from build123d import *

# Parameters (mm, degrees)
SKETCH1_W                      = 50
SKETCH1_H                      = 200
BOSS_EXTRUDE1_DEPTH            = 70
M6_CLEARANCE_HOLE1_D           = 6.6
M6_CLEARANCE_HOLE1_DEPTH       = 3.017159957
M6_CLEARANCE_HOLE1_CSINK_D     = 6.65
M6_CLEARANCE_HOLE1_CSINK_ANGLE = 100
M6_CLEARANCE_HOLE1_TIP         = 1.982840043
SKETCH5_R                      = 10
SKETCH5_R_2                    = 18.5
CUT_EXTRUDE1_DEPTH             = 40
M6_CLEARANCE_HOLE2_D           = 6.6
M6_CLEARANCE_HOLE2_CSINK_D     = 6.65
M6_CLEARANCE_HOLE2_CSINK_ANGLE = 100


with BuildPart() as part:
    # Sketch1 → Boss-Extrude1 (new body)
    with BuildSketch(Plane(origin=(0, 0, 0), x_dir=(1, 0, 0), z_dir=(0, 1, 0))):
        Rectangle(SKETCH1_W, SKETCH1_H)
    extrude(amount=BOSS_EXTRUDE1_DEPTH)

    # M6 Clearance Hole1
    with Locations(Plane(origin=(0, 0, 0), x_dir=(-1, 0, 0), z_dir=(0, -1, 0))):
        with Locations((0, 75), (0, 0), (0, -75)):
            CounterSinkHole(M6_CLEARANCE_HOLE1_D / 2, M6_CLEARANCE_HOLE1_CSINK_D / 2, depth=M6_CLEARANCE_HOLE1_DEPTH, counter_sink_angle=M6_CLEARANCE_HOLE1_CSINK_ANGLE)
            with Locations((0, 0, -(M6_CLEARANCE_HOLE1_DEPTH + M6_CLEARANCE_HOLE1_TIP / 2))):  # 118° drill point
                Cone(0, M6_CLEARANCE_HOLE1_D / 2, M6_CLEARANCE_HOLE1_TIP, mode=Mode.SUBTRACT)

    # Sketch5 → Cut-Extrude1 (cut)
    with BuildSketch(Plane.ZY.offset(25)):
        with Locations((-60, 40)):
            Circle(SKETCH5_R)
        with Locations((60, 40)):
            Circle(SKETCH5_R)
        with Locations((0, 40)):
            Circle(SKETCH5_R_2)
    extrude(amount=-CUT_EXTRUDE1_DEPTH, mode=Mode.SUBTRACT)

    # M6 Clearance Hole2 (through all)
    with Locations(Plane(origin=(0, 70, 0), x_dir=(1, 0, 0), z_dir=(0, 1, 0))):
        with Locations((-15, 40), (15, 40), (-15, -40), (15, -40)):
            CounterSinkHole(M6_CLEARANCE_HOLE2_D / 2, M6_CLEARANCE_HOLE2_CSINK_D / 2, counter_sink_angle=M6_CLEARANCE_HOLE2_CSINK_ANGLE)


solid = part.part
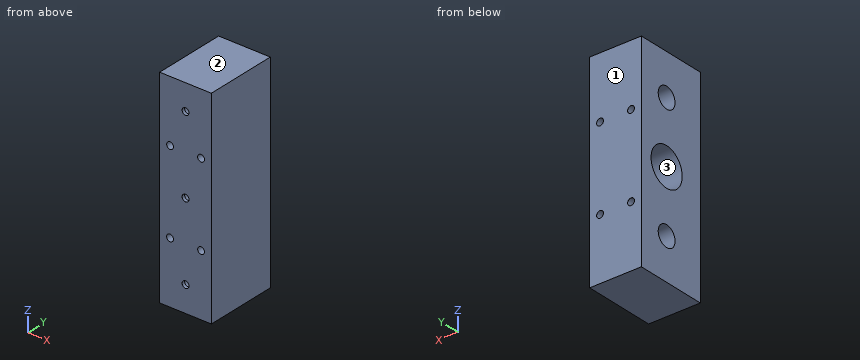
Work out the finished part from the listing and answer in its coordinate system (mm). Face numbers are marked on the shaded views. Give positions to 0.01 mm unless a question says otherwise; leave off trailing zeros. Write each loop counter-clockwise with the first axis right and the second up, starting at its lowest first coordinate (ties: lowest second). Pieces come first, ordered by that corner, then holes. Notation, with made-up numbers: M -4.75,80 L 46.25,80 A36 cw 46.25,119 Z; hole C 61.25,77.25 d4. An arc over 180 degrees is marked long. Answer as CSV lines item,"result".
Q1. Find the intervals of material crossed by probe 1 along X at (y, z) = (46, -40); probe 2 along Z at (x, y) = (0, 2); probe 3 along X at (y, z) = (63.5, -42), in increasing order. Write a range as [from, to].
A:
probe 1,"x = [-25, -18.3], [-11.7, 11.7], [18.3, 25]"
probe 2,"z = [-100, -78.3], [-71.7, -3.3], [3.3, 71.7], [78.3, 100]"
probe 3,"x = [-25, -17.62], [-12.38, 12.38], [17.62, 25]"
Q2. The mould has two halves that part along Z. Classify the marked faces 1, 2 and 3: +Z half, -Z half, draft (parallel to the pull), parting line (faces both ways), or undercut.
A:
face 1,"draft"
face 2,"+Z half"
face 3,"undercut"
Q3. A cutting plane is placed at A-A on z = -40. Write down the section's boundary in (x, y) (3 decimals).
A:
outline,"M -25,0 L -18.3,0 L -18.3,69.979 L -18.325,70 L -25,70 Z; M -11.7,0 L 11.7,0 L 11.7,69.979 L 11.675,70 L -11.675,70 L -11.7,69.979 Z; M 18.3,0 L 25,0 L 25,70 L 18.325,70 L 18.3,69.979 Z"
Q4. Given P1, Ø18, axis at y = 40, z = 60, coming from the -X side, flat-ended and moving along its own axis, determine where the tip first touches the part or whether it passes through.
A:
P1,"stops at x = 15"
Q5. A cutting plane is placed at D-D on x = -16. Count the separate pieces of the cut face and the enclosed holes in it, plus the area to 3 significant figures.
A:
separate pieces,"3"
enclosed holes,"3"
area,"11,400 mm²"
Q6. A cutting plane is placed at B-B on y = 40. Write down the section's boundary in (x, z), plus the area to 3 significant figures.
A:
outline,"M -25,-100 L 25,-100 L 25,100 L -25,100 L -25,70 L 15,70 L 15,50 L -25,50 L -25,18.5 L 15,18.5 L 15,-18.5 L -25,-18.5 L -25,-50 L 15,-50 L 15,-70 L -25,-70 Z; hole C -15,-40 d6.6; hole C -15,40 d6.6; hole C 15,-40 d6.6; hole C 15,40 d6.6"
area,"6,780 mm²"
Q7. A cutting plane is placed at C-C on z = 60. Write down the section's boundary in (x, y), plus the area to 3 significant figures.
A:
outline,"M -25,0 L 25,0 L 25,70 L -25,70 L -25,50 L 15,50 L 15,30 L -25,30 Z"
area,"2,700 mm²"
